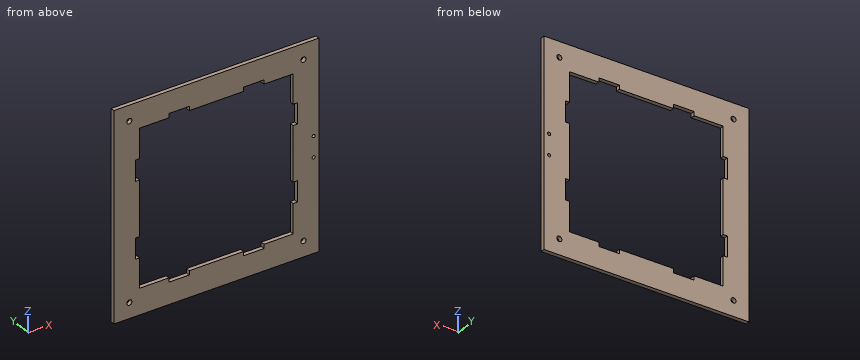
```python
from build123d import *

# Parameters (mm, degrees)
CROQUIS1_W              = 200
CROQUIS1_H              = 200
CROQUIS1_R              = 2.5
SALIENTE_EXTRUIR1_DEPTH = 4
CROQUIS2_W              = 150
CROQUIS2_H              = 150
CROQUIS2_W_2            = 4
CROQUIS2_H_2            = 20
CROQUIS2_W_3            = 20
CROQUIS2_H_3            = 4
CORTAR_EXTRUIR1_DEPTH   = 4
CROQUIS3_R              = 1.5
CORTAR_EXTRUIR2_DEPTH   = 10


with BuildPart() as part:
    # Croquis1 → Saliente-Extruir1 (new body)
    with BuildSketch(Plane(origin=(0, 0, 0), x_dir=(1, 0, 0), z_dir=(0, 1, 0))):
        with Locations((100, 100)):
            Rectangle(CROQUIS1_W, CROQUIS1_H)
        with Locations(Location((15, 185, 0), (0, 0, 270))):
            Circle(CROQUIS1_R, mode=Mode.SUBTRACT)
        with Locations(Location((185, 185, 0), (0, 0, 270))):
            Circle(CROQUIS1_R, mode=Mode.SUBTRACT)
        with Locations(Location((185, 15, 0), (0, 0, 270))):
            Circle(CROQUIS1_R, mode=Mode.SUBTRACT)
        with Locations(Location((15, 15, 0), (0, 0, 270))):
            Circle(CROQUIS1_R, mode=Mode.SUBTRACT)
    extrude(amount=SALIENTE_EXTRUIR1_DEPTH)

    # Croquis2 → Cortar-Extruir1 (cut)
    with BuildSketch(Plane(origin=(0, 4, 0), x_dir=(1, 0, 0), z_dir=(0, 1, 0))):
        with Locations((100, 100)):
            Rectangle(CROQUIS2_W, CROQUIS2_H)
        with Locations((23, 136.5)):
            Rectangle(CROQUIS2_W_2, CROQUIS2_H_2)
        with Locations((63.5, 177)):
            Rectangle(CROQUIS2_W_3, CROQUIS2_H_3)
        with Locations((177, 136.5)):
            Rectangle(CROQUIS2_W_2, CROQUIS2_H_2)
        with Locations((136.5, 177)):
            Rectangle(CROQUIS2_W_3, CROQUIS2_H_3)
        with Locations((136.5, 23)):
            Rectangle(CROQUIS2_W_3, CROQUIS2_H_3)
        with Locations((177, 63.5)):
            Rectangle(CROQUIS2_W_2, CROQUIS2_H_2)
        with Locations((23, 63.5)):
            Rectangle(CROQUIS2_W_2, CROQUIS2_H_2)
        with Locations((63.5, 23)):
            Rectangle(CROQUIS2_W_3, CROQUIS2_H_3)
    extrude(amount=-CORTAR_EXTRUIR1_DEPTH, mode=Mode.SUBTRACT)

    # Croquis3 → Cortar-Extruir2 (cut)
    with BuildSketch(Plane(origin=(0, 4, 0), x_dir=(1, 0, 0), z_dir=(0, 1, 0))):
        with Locations(Location((195, 110, 0), (0, 0, 270))):
            Circle(CROQUIS3_R)
        with Locations(Location((195, 90, 0), (0, 0, 270))):
            Circle(CROQUIS3_R)
    extrude(amount=-CORTAR_EXTRUIR2_DEPTH, mode=Mode.SUBTRACT)


solid = part.part
```
Read the model definition and answer for the solid it produces. Units are mm, in the model's axes. Coordinates: 2 decimals unless noted, no trailing zeros. Write each loop counter-clockwise with the first axis right and the second up, starting at its lowest first coordinate (ties: lowest second). Pieces come first, ordered by that corner, then holes. Notation, with made-up numbers: (-22.75, -24.5) -> (24.25, -24.5) arc R20 ccw to (24.25, 0.5) -> close; hole circle Ø5 at (35.5, 58). An arc over 180 degrees is marked (long way). Answer as a JSON object with one key per item and string values.
Q1. The part is cut by section A-A on z = -15. Give the vertices of the cut face in (x, y).
The answers:
{"outline": "(0, 0) -> (12.5, 0) -> (12.5, 4) -> (0, 4) -> close; (17.5, 0) -> (182.5, 0) -> (182.5, 4) -> (17.5, 4) -> close; (187.5, 0) -> (200, 0) -> (200, 4) -> (187.5, 4) -> close"}
Q2. The part is cut by section C-C on z = -83. Give the vertices of the cut face in (x, y), then the cut area to 3 significant figures.
The answers:
{"outline": "(0, 0) -> (25, 0) -> (25, 4) -> (0, 4) -> close; (175, 0) -> (200, 0) -> (200, 4) -> (175, 4) -> close", "area": "200 mm2"}
Q3. The part is cut by section D-D on x = 169.5. Give the vertices of the cut face in (y, z).
The answers:
{"outline": "(0, -200) -> (4, -200) -> (4, -175) -> (0, -175) -> close; (0, -25) -> (4, -25) -> (4, 0) -> (0, 0) -> close"}
Q4. Consider line 1 (X direction, y = 1.05, z = -15); line 2 (X direction, y = 2.4, z = -90); line 3 (Z direction, x = 195, y = 2.75). Determine where each line is inside the solid, lowest interval first. Write a range as [from, to].
The answers:
{"line 1": "x = [0, 12.5], [17.5, 182.5], [187.5, 200]", "line 2": "x = [0, 25], [175, 193.5], [196.5, 200]", "line 3": "z = [-200, -111.5], [-108.5, -91.5], [-88.5, 0]"}
Q5. The part is cut by section B-B on x = 15. Give the vertices of the cut face in (y, z).
The answers:
{"outline": "(0, -200) -> (4, -200) -> (4, -187.5) -> (0, -187.5) -> close; (0, -182.5) -> (4, -182.5) -> (4, -17.5) -> (0, -17.5) -> close; (0, -12.5) -> (4, -12.5) -> (4, 0) -> (0, 0) -> close"}
